Can you work these out from the model? Positions are in its coordinate system, mm. A direction names the side the tool comes from. Round coordinates to 2 decimals unless told otherwise and drop trailing zeros. Loops run counter-clockwise (first coordinate to the right, second up) from the corner with the lowest first, then second, coordinate; pieces in that order, holes last.
from build123d import *

# Parameters (mm, degrees)
EXTRUDE_THIN1_DEPTH = 25.4


with BuildPart() as part:
    # Sketch2 → Extrude-Thin1 (new body, symmetric)
    with BuildSketch(Plane(origin=(1981.2, 0, 0), x_dir=(0, 0, -1), z_dir=(1, 0, 0))):
        with BuildLine():
            Line((220.466063539, 151.267804305), (176.948936788, 218.39459013))
            ThreePointArc((176.948936788, 218.39459013), (167.722867176, 224.105285456), (157.452600901, 220.60470947))
            ThreePointArc((157.452600901, 220.60470947), (138.741359143, 55.545453365), (297.061605662, 5.252629462))
            ThreePointArc((297.061605662, 5.252629462), (304.44942683, 13.199484184), (303.002052812, 23.952972457))
            Line((303.002052812, 23.952972457), (274.455306754, 67.987389518))
            Line((274.455306754, 67.987389518), (272.32398896, 66.605693293))
            Line((272.32398896, 66.605693293), (300.870735018, 22.571276232))
            ThreePointArc((300.870735018, 22.571276232), (302.028634232, 13.968485614), (296.118377298, 7.611001836))
            ThreePointArc((296.118377298, 7.611001836), (140.872676937, 56.927149591), (159.220550284, 218.780989377))
            ThreePointArc((159.220550284, 218.780989377), (167.436763304, 221.581450166), (174.817618993, 217.012893905))
            Line((174.817618993, 217.012893905), (218.334745745, 149.88610808))
            Line((218.334745745, 149.88610808), (220.466063539, 151.267804305))
        make_face()
    extrude(amount=EXTRUDE_THIN1_DEPTH, both=True)


solid = part.part
(1) If we section it at C-C, the plane x = 1974: List the corners of the cut face in (y, z) for me.
Worked answers:
outline: (5.25, -297.06) arc R12.7 ccw to (23.95, -303) - (67.99, -274.46) - (66.61, -272.32) - (22.57, -300.87) arc R10.16 cw to (7.61, -296.12) arc R128.25 cw to (218.78, -159.22) arc R10.16 cw to (217.01, -174.82) - (149.89, -218.33) - (151.27, -220.47) - (218.39, -176.95) arc R12.7 ccw to (220.6, -157.45) arc R130.79 ccw to start
(2) If we section it at D-D, the plane y = 90: List the corners of the cut face in (x, z) for me.
Worked answers:
outline: (1955.8, -125.6) - (2006.6, -125.6) - (2006.6, -122.95) - (1955.8, -122.95) - close
(3) If I drill on line 1 (Z direction, x = 1961.5, y = 35.5); line 2 (Z direction, x = 1995.5, y = 42); line 3 (Y direction, x = 1997.5, z = -190), over which ranges is the centre line in solid material (lowest first)?
Worked answers:
line 1: z = -295.52 to -292.49, -158.31 to -154.73
line 2: z = -291.3 to -288.28, -152.18 to -148.82
line 3: y = 9.71 to 12.55, 193.59 to 198.26
(4) If we mould it in two halves opening along Y, with no side actions, what happens to faces 1 (the flat face through (2006.6, 153, -218)), 2 (the cylindrical face through (1981.556, 224.087, -167.879)), 3 (the cylindrical face through (1981.556, 57.673, -137.391)), 4 (the flat face through (1981.556, 44.897, -286.398))? For each: released by +Y, released by -Y, zero draft, split by the parting line, or undercut.
Worked answers:
face 1: zero draft
face 2: released by +Y
face 3: split by the parting line
face 4: undercut
(5) If we section it at A-A, the plane y = 157.5: List the corners of the cut face in (x, z) for me.
Worked answers:
outline: (1955.8, -216.43) - (2006.6, -216.43) - (2006.6, -213.4) - (1955.8, -213.4) - close; (1955.8, -123.99) - (2006.6, -123.99) - (2006.6, -121.38) - (1955.8, -121.38) - close
(6) Will these pins go through, and if not, where does the flat tip stop? P1, Ø6, axis at x = 2001.5, y = 175, coming from the +Z side; P2, Ø1, axis at x = 1965, z = -151.5, coming from the -Y side; P3, Ø5, axis at x = 1979.5, y = 158.5, coming from the +Z side.
Worked answers:
P1: stops at z = -125.79
P2: stops at y = 38.4
P3: stops at z = -121.02
(7) If we section it at B-B, the plane z = -153: List the corners of the cut face in (x, y) for me, then the cut area to 3 significant figures.
Worked answers:
outline: (1955.8, 37.32) - (2006.6, 37.32) - (2006.6, 41.08) - (1955.8, 41.08) - close; (1955.8, 212.31) - (2006.6, 212.31) - (2006.6, 216.07) - (1955.8, 216.07) - close
area: 382 mm2
(8) For faces 5 (the flat face through (1981.56, 183.92, -196.27)), 6 (the flat face through (1955.8, 153, -218)), which set-ups out of +Z, -Z, +X, -X, +Y, -Y let a thin tool reach every point of the face, with its end or its side?
Worked answers:
face 5: +X, -X
face 6: +Z, -Z, -X, +Y, -Y
